```python
from build123d import *

# Parameters (mm, degrees)
F0_W     = 150
F0_H     = 96.499916
F1_DEPTH = 25
F3_DEPTH = 12.5
F4_R     = 1.9
F6_DEPTH = 25
F7_R     = 7.381343
F8_DEPTH = 50


with BuildPart() as f1:
    # F0 (on Top) → F1 (new body)
    with BuildSketch(Plane.XY):
        with Locations((-75, 48.249958)):
            Rectangle(F0_W, F0_H)
    extrude(amount=F1_DEPTH)

    # F2 (on face) → F3 (intersect, symmetric)
    with BuildSketch(Plane.XY.offset(25)):
        with BuildLine():
            ThreePointArc((-43.952633, 0), (-31.079205, 31.079205), (0, 43.952633))
            Line((0, 43.952633), (0, 96.499916))
            Line((0, 96.499916), (-150, 96.499916))
            Line((-150, 96.499916), (-150, 0))
            Line((-150, 0), (-43.952633, 0))
        make_face()
    extrude(amount=F3_DEPTH, both=True, mode=Mode.INTERSECT)

    # F4
    f4_edges = [f1.edges().sort_by_distance(p)[0] for p in [
        (0, 70.226275, 25),
        (-31.079205, 31.079205, 25),
        (-96.976317, 0, 25),
        (-150, 48.249958, 25),
        (-75, 96.499916, 25),
    ]]
    fillet(f4_edges, radius=F4_R)

    # F5 (on face) → F6 (join)
    with BuildSketch(Plane.XY.offset(25)):
        Polygon((-80.540083, 24.616941), (-80.540083, 3.653123), (-60.602307, -2.825054), (-48.280083, 14.135032), (-60.602307, 31.095118), align=None)
    extrude(amount=F6_DEPTH)

    # F7 (on face) → F8 (cut)
    with BuildSketch(Plane.XY.offset(50)):
        with Locations((-67.068137, 14.832954)):
            Circle(F7_R)
    extrude(amount=-F8_DEPTH, mode=Mode.SUBTRACT)


solid = f1.part
```
Work out the finished part from the listing and answer in its coordinate system (mm). A direction names the side the tool comes from. Coordinates: 2 decimals unless noted, no trailing zeros. Loops run counter-clockwise (first coordinate to the right, second up) from the corner with the lowest first, then second, coordinate; pieces in that order, holes last.
1) Consider probe 1 along Y at (x, z) = (-82.5, 19.5); probe 2 along Z at (x, y) = (-107, 5.5); probe 3 along X at (y, z) = (14, 35). Determine where each line is inside the solid, lowest interval first.
Results:
probe 1: y = 0 to 96.5
probe 2: z = 12.5 to 25
probe 3: x = -80.54 to -74.4, -59.73 to -48.38
2) Section D-D (z = 21.5) is taken. Give the vertices of the cut face in (x, y).
Results:
outline: (-150, 0) - (-43.95, 0) arc R43.95 cw to (0, 43.95) - (0, 96.5) - (-150, 96.5) - close; hole circle Ø14.76 at (-67.07, 14.83)
3) For a pull along X with two mould halves and no side action, classify faces 1 (the flat face through (-64, 1, 25)), 2 (the flat face through (-80.54, 14, 37)), 3 (the flat face through (-54.527, 5.536, 37.325)), 4 (the flat face through (-65, 7, 50)) as +X half, -X half, draft (parallel to the pull), parting line (faces both ways), or undercut.
Results:
face 1: undercut
face 2: -X half
face 3: +X half
face 4: draft
4) Flat-ended cylindrical pins translate along their axes: pin 1 (10 mm diameter, centred on y = 71, z = 27.5, fed in from -X); pin 2 (10 mm diameter, centred on x = -89, z = 27, fed in from -Y); pin 3 (5 mm diameter, centred on y = 25.5, z = 33.5, fed in from -X). Find the tip coordinate at first contact, or state that the pin passes through.
Results:
pin 1: stops at x = -150
pin 2: stops at y = 0
pin 3: stops at x = -80.54
5) Section C-C (x = -136.5) is taken. Give the vertices of the cut face in (y, z), plus the area to 3 significant figures.
Results:
outline: (0, 12.5) - (96.5, 12.5) - (96.5, 23.1) arc R1.9 ccw to (94.6, 25) - (1.9, 25) arc R1.9 ccw to (0, 23.1) - close
area: 1,200 mm2
6) Section B-B (z = 46) is taken. Give the vertices of the cut face in (x, y).
Results:
outline: (-80.54, 3.65) - (-60.6, -2.83) - (-48.28, 14.14) - (-60.6, 31.1) - (-80.54, 24.62) - close; hole circle Ø14.76 at (-67.07, 14.83)
7) Section A-A (y = 50.5) is taken. Give the vertices of the cut face in (x, z).
Results:
outline: (-150, 12.5) - (0, 12.5) - (0, 23.1) arc R1.9 ccw to (-1.9, 25) - (-148.1, 25) arc R1.9 ccw to (-150, 23.1) - close
8) For faces 5 (the flat face through (-54.355, 22.496, 37.325)), 6 (the cylindrical face through (-60.25, 12.01, 31.51)), 7 (the flat face through (-76, 49, 12.5)), 8 (the flat face through (-70.71, 0.46, 37.33)), 9 (the flat face through (-70.43, 27.9, 37.33)), determine the directions among +Z, -Z, +X, -X, +Y, -Y from which every point of the face is accessible in a straight line to the end or side of a thin tool.
Results:
face 5: +Z, +X, +Y
face 6: +Z, -Z
face 7: -Z, +X, -X, +Y, -Y
face 8: +Z, -X, -Y
face 9: +Z, -X, +Y
